Part print with two shaded views. Sizes in mm from the minimum x, y, z corner. A direction names the side the tool comes from. Round coordinates to 2 decimals unless told otherwise and drop trailing zeros. Write each loop counter-clockwise with the first axis right and the second up, starting at its lowest first coordinate (ties: lowest second). Pieces come first, ordered by that corner, then holes. Notation, with made-up numbers: (66, -35.5) - (79, -35.5) arc R30 ccw to (79, -13.5) - close; hole circle Ø4 at (7, 75). An arc over 180 degrees is marked (long way). Use one line per item in the form item = value. Start each with the question number.
Item 1: Band-saw the part on D-D, the plane y = 15. List the corners of the cut face in (x, z), and give its area (3 significant figures).
Item 2: Band-saw the part on C-C, the plane x = 5. List the corners of the cut face in (y, z).
Item 3: Tool access for the marked faces 5, 6 and 7: list every direction of +Z, -Z, +X, -X, +Y, -Y with a clear straight run to the whole face (end or side of a thin tool).
Item 4: Band-saw the part on B-B, the plane y = 10. List the corners of the cut face in (x, z).
Item 5: Band-saw the part on A-A, the plane z = 5. List the corners of the cut face in (x, y).
Item 6: Drill centre lines: L1, parallel to X at y = 10, z = 6.85; L2, parallel to Y at x = 5, z = 7.4; L3, parallel to X at y = 5, z = 6.5. Where is each one in solid material? Low to high.
Item 7: Pin check, flat tips, straight feed: pin 1 (2 mm diameter, centred on x = 15, y = 15, fed in from +Z); pin 2 (4 mm diameter, centred on y = 17, z = 7, fed in from -X); pin 3 (5 mm diameter, centred on x = 14.5, z = 6, fed in from -Y); pin 4 (6 mm diameter, centred on x = 5, y = 10, fed in from +Z). Stop position of each tip, or through.
Item 8: Pull direction Y, two halves, no side cores. Call the marked faces 1, 2, 3 and 4: +Y half, -Y half, draft (parallel to the pull), parting line (faces both ways), or undercut.
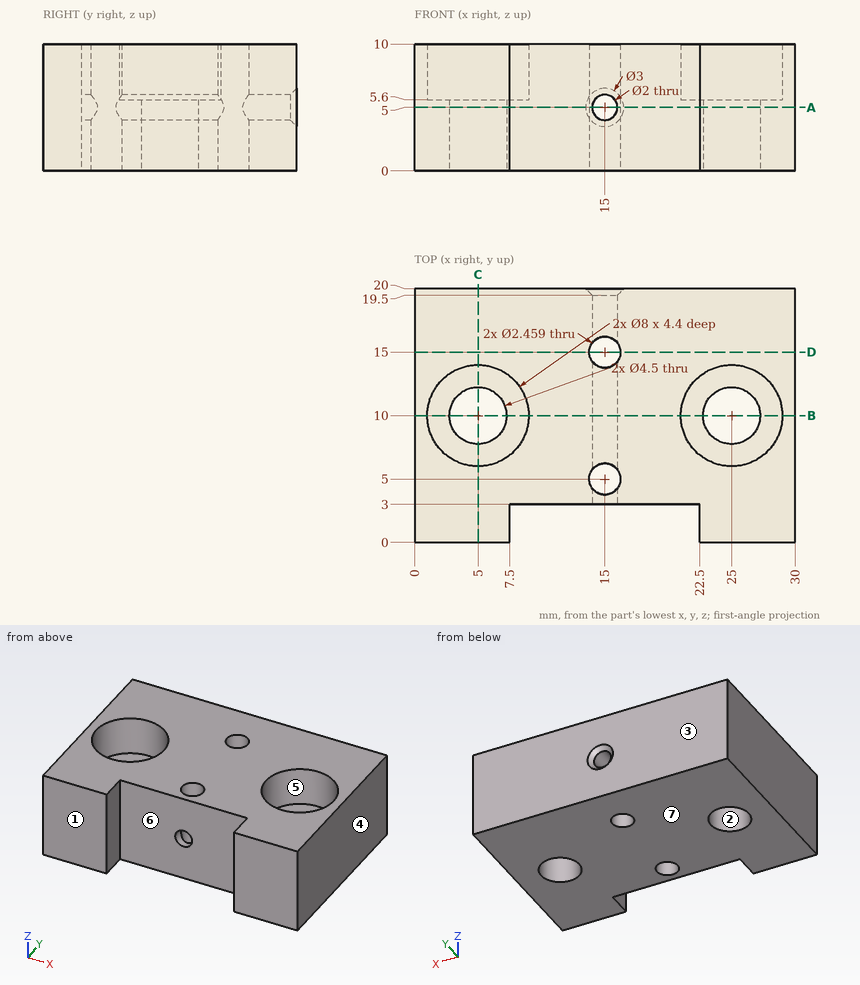
Determined:
q1.outline = (0, 0) - (13.77, 0) - (13.77, 10) - (0, 10) - close; (16.23, 0) - (30, 0) - (30, 10) - (16.23, 10) - close
q1.area = 275 mm²
q2.outline = (0, 0) - (7.75, 0) - (7.75, 5.6) - (6, 5.6) - (6, 10) - (0, 10) - close; (12.25, 0) - (20, 0) - (20, 10) - (14, 10) - (14, 5.6) - (12.25, 5.6) - close
q3.face_5 = +Z
q3.face_6 = +Z, -Z, -Y
q3.face_7 = -Z, +X, -X, +Y, -Y
q4.outline = (0, 0) - (2.75, 0) - (2.75, 5.6) - (1, 5.6) - (1, 10) - (0, 10) - close; (7.25, 0) - (22.75, 0) - (22.75, 5.6) - (21, 5.6) - (21, 10) - (9, 10) - (9, 5.6) - (7.25, 5.6) - close; (27.25, 0) - (30, 0) - (30, 10) - (29, 10) - (29, 5.6) - (27.25, 5.6) - close; hole circle Ø2 at (15, 5)
q5.outline = (0, 0) - (7.5, 0) - (7.5, 3) - (14, 3) - (14, 4.28) arc R1.23 cw to (14, 5.72) - (14, 14.28) arc R1.23 cw to (14, 15.72) - (14, 19.5) - (13.5, 20) - (0, 20) - close; (16, 3) - (22.5, 3) - (22.5, 0) - (30, 0) - (30, 20) - (16.5, 20) - (16, 19.5) - (16, 15.72) arc R1.23 cw to (16, 14.28) - (16, 5.72) arc R1.23 cw to (16, 4.28) - close; hole circle Ø4.5 at (5, 10); hole circle Ø4.5 at (25, 10)
q6.L1 = 0 to 1, 9 to 21, 29 to 30
q6.L2 = 0 to 6, 14 to 20
q6.L3 = 0 to 13.77, 16.23 to 30
q7.pin_1 = through
q7.pin_2 = 0
q7.pin_3 = 3
q7.pin_4 = 5.6
q8.face_1 = -Y half
q8.face_2 = undercut
q8.face_3 = +Y half
q8.face_4 = draft
